The model under review builds one solid part; all positions refer to its coordinate system, in mm. A direction names the side the tool comes from. Give positions to 0.01 mm unless a question says otherwise; leave off trailing zeros. Order: outer loops, then holes, each group sorted by start corner. A loop starts at its lowest first (then second) coordinate and runs counter-clockwise, first axis right, second up. Notation, with made-up numbers: M 32.5,5 L 69.5,5 A23 ccw 69.5,38 Z; hole C -31,-4.75 d10. An arc over 180 degrees is marked long. One line per question, with ' | ' between items. Start each with the question number.
1. We need section A-A on z = 32. Write out the cut boundary in (x, y), then the cut area to 3 significant figures.
2. We need section D-D on x = 33. Write out the cut boundary in (y, z).
3. We need section C-C on y = -13. Write out the cut boundary in (x, z).
4. The part is to be moulded in two halves that separate along X. For faces 4 (the face through (-9.068, 4, 32)), 5 (the face through (94.721, -8.112, 56.028)), 6 (the face through (134.932, -1, 32)), 7 (the face through (78, -4, 64)), say which applies: +X half, -X half, draft (parallel to the pull), parting line (faces both ways), or undercut.
5. We need section B-B on x = 1.5. Write out the cut boundary in (y, z), then the cut area to 3 significant figures.
6. For faces 1 (the face through (49, -12, 48)), 2 (the face through (2, 20, 24)), 3 (the face through (2, 36, 32)), list the 3-axis set-ups (+Z, -Z, +X, -X, +Y, -Y) from which the entire face can be reached by the end or side of a thin tool; tool diameter is ignored.
7. Insertion check: P1, Ø3, axis at x = 111.5, z = 35, coming from the +Y side; P2, Ø9.5, axis at x = 96.93, z = 54, coming from the +Y side; P3, Ø2, axis at x = 10.5, z = 35, coming from the +Y side; P4, Ø2, axis at x = 98.5, z = 55, coming from the +Y side. Each pin has a flat end and moves straight along its axis. Give the tip position at first contact, or say it passes through.
8. Wall thickness on L1, parallel to X at y = 7, z = 17; L2, parallel to Y at x = 1, z = 32; L3, parallel to Z at x = 79, y = -8: over which ranges is each line inside the solid? List them lowest first.
Autodesk Inventor part; units mm, degrees
ref_plane "YZ Plane" through (0, 0, 0) normal (1, 0, 0) x (0, 1, 0)
ref_plane "XZ Plane" through (0, 0, 0) normal (0, 1, 0) x (-1, 0, 0)
ref_plane "XY Plane" through (0, 0, 0) normal (0, 0, 1) x (1, 0, 0)
sketch "Sketch1" plane through (0, 0, 0) normal (0, 0, 1) x (1, 0, 0)
  line L0 (12.9321, 0) -> (108.9321, 0)
  line L1 (108.9321, -16) -> (-9.0679, -16)
  line L2 (-9.0679, -16) -> (-9.0679, 0)
  line L3 (12.9321, 0) -> (12.9321, 36)
  line L4 (12.9321, 36) -> (-9.0679, 36)
  line L5 (-9.0679, 36) -> (-9.0679, 0)
  line L6 (108.9321, -16) -> (134.9321, -16)
  line L7 (134.9321, -16) -> (134.9321, 14)
  line L8 (108.9321, 0) -> (108.9321, 26)
  line L9 (108.9321, 26) -> (118.9321, 26)
  line L10 (118.9321, 26) -> (134.9321, 14)
  point P0 (0, 0)
  dimension "d0" = 118
  dimension "d1" = 16
  dimension "d2" = 22
  dimension "d3" = 36
  dimension "d4" = 26
  dimension "d5" = 30
  dimension "d6" = 26
  dimension "d7" = 10
extrude "Extrusion1" add sketch "Sketch1" along normal blind 64
sketch "Sketch2" plane through (-9.0679, -16, 0) normal (-1, 0, 0) x (0, 0, 1)
  circle A0 centre (32, 36) radius 8
  line L0 (0, 0) -> (64, 0)
  line L1 (0, 52) -> (0, 0)
  line L2 (0, 16) -> (64, 16)
  line L3 (0, 16) -> (4.0233, 16)
  line L4 (64, 16) -> (59.9767, 16)
  arc A1 (46.702, 42.3127) -> (17.298, 42.3127) centre (32, 36) ccw
  line L5 (57.2201, 17.8164) -> (46.702, 42.3127)
  line L6 (6.7799, 17.8164) -> (17.298, 42.3127)
  arc A2 (4.0233, 16) -> (6.7799, 17.8164) centre (4.0233, 19) ccw
  arc A3 (57.2201, 17.8164) -> (59.9767, 16) centre (59.9767, 19) ccw
  line L7 (0, 16) -> (0, 52)
  line L8 (0, 52) -> (64, 52)
  line L9 (64, 52) -> (64, 16)
  line L10 (64, 52) -> (64, 0)
  point P0 (6, 16)
  point P1 (58, 16)
  point P2 (32, 52)
  dimension "d10" = 16
  dimension "d11" = 36
  dimension "d12" = 32
  dimension "d13" = 6
  dimension "d14" = 6
  dimension "d15" = 3
  dimension "d16" = 3
extrude "Extrusion2" cut sketch "Sketch2" against normal blind 22 contours A0 | L1 L8 A1 L6 A2 L2 | L2 A3 L5 A1 L8 L9
sketch "Sketch3" plane through (-9.0679, -16, 0) normal (-1, 0, 0) x (0, 0, 1)
  line L0 (0, 0) -> (64, 0)
  line L1 (0, 16) -> (64, 16)
  line L2 (48, 0) -> (16, 0)
  line L3 (16, 0) -> (16, 7)
  line L4 (24, 16) -> (40, 16)
  line L5 (48, 7) -> (48, 0)
  line L6 (0, 16) -> (0, 0)
  line L7 (64, 16) -> (64, 0)
  line L8 (24, 16) -> (24, 7)
  line L9 (24, 7) -> (16, 7)
  line L10 (48, 7) -> (40, 7)
  line L11 (40, 7) -> (40, 16)
  point P0 (16, 0)
  dimension "d19" = 16
  dimension "d20" = 16
  dimension "d21" = 9
  dimension "d22" = 8
  dimension "d23" = 8
extrude "Extrusion3" cut sketch "Sketch3" against normal blind 118 contours L3 L9 L8 L1 L11 L10 L5 L0
sketch "Sketch4" plane through (-9.0679, -16, 0) normal (0, -1, 0) x (1, 0, 0)
  circle A0 centre (36, 54) radius 3
  line L0 (0, 48) -> (0, 64)
  line L1 (0, 64) -> (144, 64)
  circle A1 centre (106, 54) radius 3
  circle A2 centre (36, 10) radius 3
  circle A3 centre (106, 10) radius 3
  point P0 (9.0679, 0)
  dimension "d26" = 6
  dimension "d27" = 36
  dimension "d28" = 10
  dimension "d31" = 70
  dimension "d34" = 44
extrude "Extrusion4" cut sketch "Sketch4" against normal through all
properties part number "first"
Entries:
1) outline: M -9.07,0 L 12.93,0 L 12.93,12 L -9.07,12 Z; M -9.07,28 L 12.93,28 L 12.93,36 L -9.07,36 Z; M 108.93,-16 L 134.93,-16 L 134.93,14 L 118.93,26 L 108.93,26 Z | area: 1,440 mm^2
2) outline: M -16,0 L 0,0 L 0,24 L -9,24 L -9,16 L -16,16 Z; M -16,48 L -9,48 L -9,40 L 0,40 L 0,64 L -16,64 Z
3) outline: M -9.07,0 L 134.93,0 L 134.93,64 L -9.07,64 L -9.07,48 L 108.93,48 L 108.93,16 L -9.07,16 Z; hole C 26.93,10 d6; hole C 26.93,54 d6; hole C 96.93,10 d6; hole C 96.93,54 d6
4) face 4: -X half | face 5: undercut | face 6: +X half | face 7: draft
5) outline: M -16,0 L 0,0 L 0,4.02 A3 cw 1.82,6.78 L 26.31,17.3 A16 ccw 26.31,46.7 L 1.82,57.22 A3 cw 0,59.98 L 0,64 L -16,64 L -16,48 L -9,48 L -9,40 L 0,40 L 0,24 L -9,24 L -9,16 L -16,16 Z; hole C 20,32 d16 | area: 1,730 mm^2
6) face 1: -X, -Y | face 2: -X | face 3: +X, -X, +Y
7) P1: stops at y = 26 | P2: stops at y = 0 | P3: stops at y = 35.87 | P4: passes through
8) L1: x = -9.07 to 12.93, 108.93 to 134.93 | L2: y = 0 to 12, 28 to 36 | L3: z = 0 to 24, 40 to 64
